Check sheet for the drawn part. Datum: minimum x, y, z corner. Units: mm. A direction names the side the tool comes from. Give positions to 0.01 mm unless a question says otherwise; leave off trailing zeros. Loops run counter-clockwise (first coordinate to the right, second up) from the corner with the lowest first, then second, coordinate; pieces in that order, holes last. Notation, with made-up numbers: (59.5, -25.5) - (75.5, -25.5) arc R17 cw to (75.5, -7.5) - close; hole circle Ø9 at (42, 8.25). An arc over 180 degrees is marked (long way). Answer in a Markdown table with one row per item.
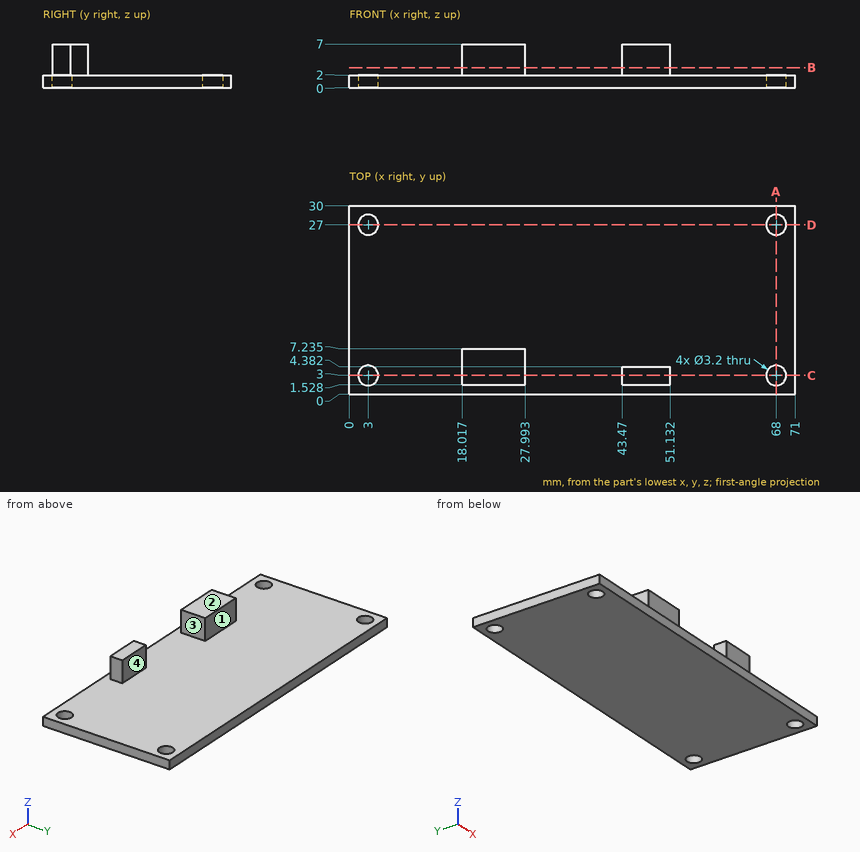
Q1. Go/stop test with flat-tipped pins: P1, Ø1, axis at y = 15.5, z = 2, coming from the -X side; P2, Ø5, axis at x = 68, y = 3, coming from the +Z side; P3, Ø2.5, axis at y = 4.5, z = 4.5, coming from the +X side; P4, Ø4, axis at x = 24, z = 5.5, coming from the -Y side. Record where each tip stops, or that it passes through.
Completed:
| item | result |
|---|---|
| P1 | x = 0 |
| P2 | z = 2 |
| P3 | x = 51.13 |
| P4 | y = 1.53 |
Q2. Draft check along X on the marked faces 3 and 4. Enter one of: +X half, -X half, draft (parallel to the pull), parting line (faces both ways), or undercut.
Completed:
| item | result |
|---|---|
| face 3 | undercut |
| face 4 | draft |
Q3. Sectioned sample at A-A (x = 68). Record the cut outline in (y, z).
Completed:
| item | result |
|---|---|
| outline | (0, 0) - (1.4, 0) - (1.4, 2) - (0, 2) - close; (4.6, 0) - (25.4, 0) - (25.4, 2) - (4.6, 2) - close; (28.6, 0) - (30, 0) - (30, 2) - (28.6, 2) - close |
Q4. Sectioned sample at B-B (z = 3.25). Record the cut outline in (x, y) (1 decimal).
Completed:
| item | result |
|---|---|
| outline | (18, 1.5) - (28, 1.5) - (28, 7.2) - (18, 7.2) - close; (43.5, 1.5) - (51.1, 1.5) - (51.1, 4.4) - (43.5, 4.4) - close |
Q5. Tool access check on the marked faces 1 and 2. Record the directions out of +Z, -Z, +X, -X, +Y, -Y that give a thin tool (end or side, any length) a straight path to the whole face; none if there is none.
Completed:
| item | result |
|---|---|
| face 1 | +Z, +X, -X, +Y |
| face 2 | +Z, +X, -X, +Y, -Y |
Q6. Sectioned sample at D-D (y = 27). Record the cut outline in (x, z), and give its area (3 significant figures).
Completed:
| item | result |
|---|---|
| outline | (0, 0) - (1.4, 0) - (1.4, 2) - (0, 2) - close; (4.6, 0) - (66.4, 0) - (66.4, 2) - (4.6, 2) - close; (69.6, 0) - (71, 0) - (71, 2) - (69.6, 2) - close |
| area | 129 mm^2 |
Q7. Thickness scan on line 1 (Y direction, x = 68, z = 0.7); line 2 (Z direction, x = 58.5, y = 9); line 3 (Y direction, x = 26, z = 3.5) (1 decimal). Record the ranges inside material, lowest first.
Completed:
| item | result |
|---|---|
| line 1 | 0 to 1.4, 4.6 to 25.4, 28.6 to 30 |
| line 2 | 0 to 2 |
| line 3 | 1.5 to 7.2 |
Q8. Sectioned sample at C-C (y = 3). Record the cut outline in (x, z).
Completed:
| item | result |
|---|---|
| outline | (0, 0) - (1.4, 0) - (1.4, 2) - (0, 2) - close; (4.6, 0) - (66.4, 0) - (66.4, 2) - (51.13, 2) - (51.13, 7) - (43.47, 7) - (43.47, 2) - (27.99, 2) - (27.99, 7) - (18.02, 7) - (18.02, 2) - (4.6, 2) - close; (69.6, 0) - (71, 0) - (71, 2) - (69.6, 2) - close |
